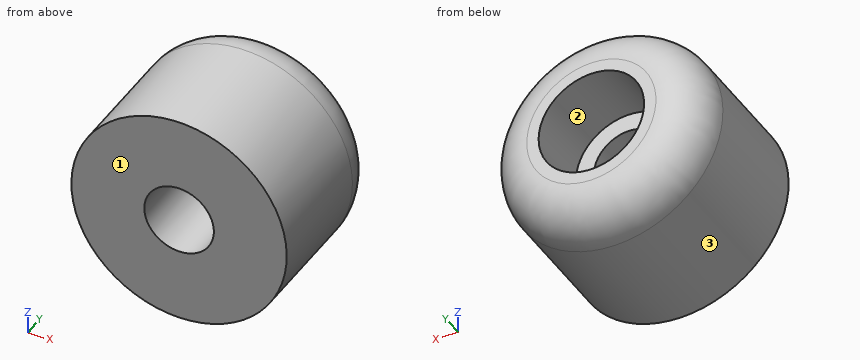
```python
from build123d import *

# Parameters (mm, degrees)
CROQUIS1_R                                           = 12.7
SALIENTE_EXTRUIR1_DEPTH                              = 19.05
REFRENTADO_PARA_TORNILLO_CON_CABEZA_HUEC_D           = 8.2042
REFRENTADO_PARA_TORNILLO_CON_CABEZA_HUEC_DEPTH       = 19.7485
REFRENTADO_PARA_TORNILLO_CON_CABEZA_HUEC_CBORE_D     = 12.446
REFRENTADO_PARA_TORNILLO_CON_CABEZA_HUEC_CBORE_DEPTH = 7.9375
REFRENTADO_PARA_TORNILLO_CON_CABEZA_HUEC_TIP         = 2.464790345
REDONDEO1_R                                          = 5.08


with BuildPart() as part:
    # Croquis1 → Saliente-Extruir1 (new body)
    with BuildSketch(Plane(origin=(0, 0, 0), x_dir=(1, 0, 0), z_dir=(0, 1, 0))):
        with Locations(Location((0, 0, 0), (0, 0, 90))):
            Circle(CROQUIS1_R)
    extrude(amount=SALIENTE_EXTRUIR1_DEPTH)

    # Refrentado para tornillo con cabeza hueca de 5/161
    with Locations(Plane(origin=(0, 19.05, 0), x_dir=(1, 0, 0), z_dir=(0, 1, 0))):
        with Locations((0, 0)):
            CounterBoreHole(REFRENTADO_PARA_TORNILLO_CON_CABEZA_HUEC_D / 2, REFRENTADO_PARA_TORNILLO_CON_CABEZA_HUEC_CBORE_D / 2, REFRENTADO_PARA_TORNILLO_CON_CABEZA_HUEC_CBORE_DEPTH, depth=REFRENTADO_PARA_TORNILLO_CON_CABEZA_HUEC_DEPTH)
            with Locations((0, 0, -(REFRENTADO_PARA_TORNILLO_CON_CABEZA_HUEC_DEPTH + REFRENTADO_PARA_TORNILLO_CON_CABEZA_HUEC_TIP / 2))):  # 118° drill point
                Cone(0, REFRENTADO_PARA_TORNILLO_CON_CABEZA_HUEC_D / 2, REFRENTADO_PARA_TORNILLO_CON_CABEZA_HUEC_TIP, mode=Mode.SUBTRACT)

    # Redondeo1
    redondeo1_edges = [part.edges().sort_by_distance(p)[0] for p in [
        (0, 19.05, 12.7),
    ]]
    fillet(redondeo1_edges, radius=REDONDEO1_R)


solid = part.part
```
Geometry: final body of the model. Coordinates: model frame, mm. Face numbers are marked on the shaded views. Coordinates: 2 decimals unless noted, no trailing zeros. Order: outer loops, then holes, each group sorted by start corner. A loop starts at its lowest first (then second) coordinate and runs counter-clockwise, first axis right, second up. Notation, with made-up numbers: (-15, 21) -> (-1, 21) arc R27 cw to (-1, 42) -> close; hole circle Ø10 at (23, 12). An arc over 180 degrees is marked (long way). Answer in a Markdown table with one row per item.
Item 1: Contact query for flat-ended pins moving along their axis: P1, Ø3, axis at x = -4, z = 1.5, coming from the +Y side; P2, Ø1.5, axis at y = 14, z = -2.5, coming from the +X side; P3, Ø2, axis at x = -7, z = 6.5, coming from the +Y side. Output: stop coordinate, or through.
Return value:
| item | result |
|---|---|
| P1 | stops at y = 11.11 |
| P2 | stops at x = 12.58 |
| P3 | stops at y = 18.96 |
Item 2: Section A-A on x = 0. Output: boundary loops of the cut face in (y, z).
Return value:
| item | result |
|---|---|
| outline | (0, -12.7) -> (13.97, -12.7) arc R5.08 ccw to (19.05, -7.62) -> (19.05, -6.22) -> (11.11, -6.22) -> (11.11, -4.1) -> (0, -4.1) -> close; (0, 4.1) -> (11.11, 4.1) -> (11.11, 6.22) -> (19.05, 6.22) -> (19.05, 7.62) arc R5.08 ccw to (13.97, 12.7) -> (0, 12.7) -> close |
Item 3: Section B-B on z = 0. Output: boundary loops of the cut face in (x, y).
Return value:
| item | result |
|---|---|
| outline | (-12.7, 0) -> (-4.1, 0) -> (-4.1, 11.11) -> (-6.22, 11.11) -> (-6.22, 19.05) -> (-7.62, 19.05) arc R5.08 ccw to (-12.7, 13.97) -> close; (4.1, 0) -> (12.7, 0) -> (12.7, 13.97) arc R5.08 ccw to (7.62, 19.05) -> (6.22, 19.05) -> (6.22, 11.11) -> (4.1, 11.11) -> close |
Item 4: Section C-C on y = 12.25. Output: boundary loops of the cut face in (x, z).
Return value:
| item | result |
|---|---|
| outline | circle Ø25.4 at (0, 0); hole circle Ø12.45 at (0, 0) |
Item 5: Section D-D on y = 4.25. Output: boundary loops of the cut face in (x, z), plus the area to 3 significant figures.
Return value:
| item | result |
|---|---|
| outline | circle Ø25.4 at (0, 0); hole circle Ø8.2 at (0, 0) |
| area | 454 mm² |
Item 6: Ray query, L1, parallel to X at y = 2.25, z = 2; L2, parallel to X at y = 3.25, z = -0.75; L3, parallel to Z at x = 0.5, y = 3. Return the intervals inside material, ascending.
Return value:
| item | result |
|---|---|
| L1 | x = -12.54 to -3.58, 3.58 to 12.54 |
| L2 | x = -12.68 to -4.03, 4.03 to 12.68 |
| L3 | z = -12.69 to -4.07, 4.07 to 12.69 |
Item 7: Draft query along X for the marked faces 1, 2 and 3. Return one class per face: released by +X, released by -X, zero draft, split by the parting line, or undercut.
Return value:
| item | result |
|---|---|
| face 1 | zero draft |
| face 2 | undercut |
| face 3 | split by the parting line |
